from build123d import *

# Parameters (mm, degrees)
F0_R     = 9.525
F0_R_2   = 3.2385
F1_DEPTH = 12.954
F2_R     = 4.1275
F3_DEPTH = 6.35
F5_R     = 1.5875
F6_DEPTH = 31.75
F7_DEPTH = 25.4
F5_R_2   = 4.445
F8_DEPTH = 17.78


with BuildPart() as f1:
    # F0 (on Top) → F1 (new body)
    with BuildSketch(Plane.XY):
        Circle(F0_R)
        Circle(F0_R_2, mode=Mode.SUBTRACT)
    extrude(amount=F1_DEPTH)

    # F2 (on face) → F3 (join)
    with BuildSketch(Plane.XY.offset(12.954)):
        with BuildLine():
            ThreePointArc((-0.3406139649, -9.5189078747), (6.6136705763, -6.8545595415), (9.525, 0))
            ThreePointArc((9.525, 0), (6.6137479521, 6.8544848841), (-0.3403990606, 9.5189155622))
            ThreePointArc((-0.3403990606, 9.5189155622), (-9.5249999994, 0.0001075209), (-0.3406139649, -9.5189078747))
        make_face()
        with BuildLine():
            ThreePointArc((-0.3406139649, -9.5189078747), (-9.5249999994, 0.0001075209), (-0.3403990606, 9.5189155622))
            Line((-0.3403990606, 9.5189155622), (-88.965388203, 6.3496633283))
            ThreePointArc((-88.965388203, 6.3496633283), (-84.4330499829, 4.5131870717), (-82.55, 0))
            ThreePointArc((-82.55, 0), (-84.4098719395, -4.4901280605), (-88.9, -6.35))
            Line((-88.9, -6.35), (-0.3406139649, -9.5189078747))
        make_face()
        with Locations((-76.581, 0)):
            Circle(F2_R, mode=Mode.SUBTRACT)
        with Locations((-64.262, 0)):
            Circle(F2_R, mode=Mode.SUBTRACT)
        with Locations((-51.943, 0)):
            Circle(F2_R, mode=Mode.SUBTRACT)
        with Locations((-39.624, 0)):
            Circle(F2_R, mode=Mode.SUBTRACT)
        with Locations((-27.305, 0)):
            Circle(F2_R, mode=Mode.SUBTRACT)
        with Locations((-14.986, 0)):
            Circle(F2_R, mode=Mode.SUBTRACT)
        with BuildLine():
            ThreePointArc((-82.55, 0), (-84.4330499829, 4.5131870717), (-88.965388203, 6.3496633283))
            ThreePointArc((-88.965388203, 6.3496633283), (-95.2499158315, -0.0326945349), (-88.9, -6.35))
            ThreePointArc((-88.9, -6.35), (-84.4098719395, -4.4901280605), (-82.55, 0))
        make_face()
        with Locations((-88.9, 0)):
            Circle(F2_R, mode=Mode.SUBTRACT)
    extrude(amount=-F3_DEPTH)

    # F5 (on offset) → F6 (cut)
    with BuildSketch(Plane.YZ.offset(25.4)):
        with Locations((0, 6.096)):
            Circle(F5_R)
    extrude(amount=-F6_DEPTH, mode=Mode.SUBTRACT)

    # F0 (on Top) → F7 (cut)
    with BuildSketch(Plane.XY):
        Circle(F0_R_2)
    extrude(amount=F7_DEPTH, mode=Mode.SUBTRACT)

    # F5 (on offset) → F8 (cut)
    with BuildSketch(Plane.YZ.offset(25.4)):
        with Locations((0, 6.096)):
            Circle(F5_R_2)
        with Locations((0, 6.096)):
            Circle(F5_R, mode=Mode.SUBTRACT)
    extrude(amount=-F8_DEPTH, mode=Mode.SUBTRACT)


solid = f1.part
The model under review builds one solid part; all positions refer to its coordinate system, in mm. A direction names the side the tool comes from. Coordinates: 2 decimals unless noted, no trailing zeros. Put each result on its own line as item: value.
1) Draft analysis for pull direction X (two halves, no side actions). For faces 1 (the flat face through (7.62, 0, 4)), 2 (the cylindrical face through (-2.57, -1.97, 6.39)), 3 (the flat face through (-32, 0, 12.954)), state which applies: released by +X, released by -X, zero draft, split by the parting line, or undercut.
Computed:
face 1: released by +X
face 2: undercut
face 3: zero draft
2) For faces 4 (the cylindrical face through (-68.386, 0.181, 9.823)), 5 (the cylindrical face through (8.374, -0.964, 1.757)), list the 3-axis set-ups (+Z, -Z, +X, -X, +Y, -Y) from which the entire face can be reached by the end or side of a thin tool; tool diameter is ignored.
Computed:
face 4: +Z, -Z
face 5: +X
3) Wall thickness on probe 1 along Y at (x, z) = (-88.9, 10); probe 2 along Y at (x, z) = (0, 12) (1 decimal); probe 3 along Z at (x, y) = (-44, -6.25): over which ranges is each line inside the solid? List them lowest first. Write a range as [from, to].
Computed:
probe 1: y = [-6.35, -4.13], [4.13, 6.35]
probe 2: y = [-9.5, -3.2], [3.2, 9.5]
probe 3: z = [6.6, 12.95]
4) Add section A-A on y = 0. State how many separate pieces and enclosed holes the cut face has, then the cut area to 3 significant figures.
Computed:
separate pieces: 10
enclosed holes: 0
area: 300 mm2
5) Clearance check with flat-ended pins moving along their axes: pin 1 Ø1 at (y, z) = (6, 5.5) entering from -X; pin 2 Ø1.5 at (y, z) = (3, 11.5) entering from -X; pin 3 Ø7.5 at (x, y) = (-27.305, 0) entering from +Z; pin 4 Ø4.5 at (y, z) = (0.5, 8) entering from +X. State where each tip first meets the part, or that it passes through.
Computed:
pin 1: stops at x = -7.78
pin 2: stops at x = -94.84
pin 3: passes through
pin 4: stops at x = 7.62
